from build123d import *

# Parameters (mm, degrees)
F1_R         = 2.5
F2_DEPTH     = 7.5
F3_W         = 3.4
F3_H         = 15.4505071864
F3_W_2       = 3.8797123611
F3_W_3       = 3.8316924378
F4_DEPTH     = 16.41578
F6_DEPTH     = 2.8
F8_DEPTH     = 2.8
F9_R         = 0.1
F10_R        = 2.5
F11_DEPTH    = 7.5
F12_W        = 3
F12_H        = 7.5577301905
F13_DEPTH    = 15.0010001
F14_T1_DEPTH = 16.5892781094
F16_W        = 15
F16_H        = 15
F17_DEPTH    = 30


# Not quite as in the source:
# - a fillet or chamfer that OpenCascade refuses, or shapes differently, is made with other operations: its cross-section is extruded or revolved along the edge and cut away or added


with BuildPart() as f2:
    # F1 (on Right) → F2 (new body, symmetric)
    with BuildSketch(Plane.YZ):
        with BuildLine():
            Line((7.5, -12.5), (7.5, 0))
            ThreePointArc((7.5, 0), (0, 7.5), (-7.5, 0))
            Line((-7.5, 0), (-7.5, -12.5))
            Line((-7.5, -12.5), (7.5, -12.5))
        make_face()
        Circle(F1_R, mode=Mode.SUBTRACT)
    extrude(amount=F2_DEPTH, both=True)

    # F3 (on Front) → F4 (cut, symmetric)
    with BuildSketch(Plane.XZ):
        with Locations((0, 0.7252535932)):
            Rectangle(F3_W, F3_H)
        with Locations((-6.6398561805, 0.7252535932)):
            Rectangle(F3_W_2, F3_H)
        with Locations((6.6158462189, 0.7252535932)):
            Rectangle(F3_W_3, F3_H)
    extrude(amount=F4_DEPTH, both=True, mode=Mode.SUBTRACT)

    # F5 (on face) → F6 (cut, through all)
    with BuildSketch(Plane(origin=(-7.5, 0, 0), x_dir=(0, -1, 0), z_dir=(-1, 0, 0))):
        with BuildLine():
            ThreePointArc((2.6925824036, -7), (6.1824092402, -4.2459175671), (7.5, 0))
            ThreePointArc((7.5, 0), (-4.2459175671, 6.1824092402), (-2.6925824036, -7))
            Line((-2.6925824036, -7), (2.6925824036, -7))
        make_face()
        with BuildLine():
            Line((2.6925824036, -7), (-2.6925824036, -7))
            ThreePointArc((-2.6925824036, -7), (0, -7.5), (2.6925824036, -7))
        make_face()
    extrude(amount=-F6_DEPTH, mode=Mode.SUBTRACT)

    # F7 (on face) → F8 (cut, through all)
    with BuildSketch(Plane.YZ.offset(7.5)):
        with BuildLine():
            Line((2.6925824036, -7), (-2.6925824036, -7))
            ThreePointArc((-2.6925824036, -7), (0, -7.5), (2.6925824036, -7))
        make_face()
        with BuildLine():
            ThreePointArc((2.6925824036, -7), (6.1824092402, -4.2459175671), (7.5, 0))
            ThreePointArc((7.5, 0), (-4.2459175671, 6.1824092402), (-2.6925824036, -7))
            Line((-2.6925824036, -7), (2.6925824036, -7))
        make_face()
    extrude(amount=-F8_DEPTH, mode=Mode.SUBTRACT)

    # F9
    f9_edges = [f2.edges().sort_by_distance(p)[0] for p in [
        (7.5, -5.096291, -7),
        (7.5, 0, -7.5),
        (7.5, 5.096291, -7),
        (-7.5, 5.096291, -7),
        (-7.5, 0, -7.5),
        (-7.5, -5.096291, -7),
    ]]
    fillet(f9_edges, radius=F9_R)

    # F16 (on face) → F17 (join)
    with BuildSketch(Plane(origin=(0, 0, -12.5), x_dir=(1, 0, 0), z_dir=(0, 0, -1))):
        Rectangle(F16_W, F16_H)
    extrude(amount=F17_DEPTH)

    # F18: F2 across face


with BuildPart() as f11:
    # F10 (on Right) → F11 (new body, symmetric)
    with BuildSketch(Plane.YZ):
        with BuildLine():
            Line((-7.5, 15.0892781094), (-7.5, 0))
            ThreePointArc((-7.5, 0), (0, -7.5), (7.5, 0))
            Line((7.5, 0), (7.5, 15.0892781094))
            Line((7.5, 15.0892781094), (-7.5, 15.0892781094))
        make_face()
        Circle(F10_R, mode=Mode.SUBTRACT)
    extrude(amount=F11_DEPTH, both=True)

    # F12 (on face) → F13 (cut, through all)
    with BuildSketch(Plane.XZ.offset(7.5)):
        with Locations((-3.2, 3.7788650952)):
            Rectangle(F12_W, F12_H)
        with Locations((3.2, 3.7788650952)):
            Rectangle(F12_W, F12_H)
    extrude(amount=-F13_DEPTH, mode=Mode.SUBTRACT)

    # F14: fillet of radius 0.1 on 4 edges, made by hand

    # F14_s2 → F14_t1 (cut)
    with BuildSketch(Plane.XY.offset(-1.25)):
        with BuildLine():
            ThreePointArc((-7.4, 7.5), (-7.4707106781, 7.4707106781), (-7.5, 7.4))
            Line((-7.5, 7.4), (-7.5, 7.5))
            Line((-7.5, 7.5), (-7.4, 7.5))
        make_face()
        with BuildLine():
            ThreePointArc((-7.5, -7.4), (-7.4707106781, -7.4707106781), (-7.4, -7.5))
            Line((-7.4, -7.5), (-7.5, -7.5))
            Line((-7.5, -7.5), (-7.5, -7.4))
        make_face()
        with BuildLine():
            ThreePointArc((7.4, 7.5), (7.4707106781, 7.4707106781), (7.5, 7.4))
            Line((7.5, 7.4), (7.5, 7.5))
            Line((7.5, 7.5), (7.4, 7.5))
        make_face()
        with BuildLine():
            ThreePointArc((7.5, -7.4), (7.4707106781, -7.4707106781), (7.4, -7.5))
            Line((7.4, -7.5), (7.5, -7.5))
            Line((7.5, -7.5), (7.5, -7.4))
        make_face()
    extrude(amount=F14_T1_DEPTH, mode=Mode.SUBTRACT)


with BuildPart() as f2_1:
    add(f2.part)
    add(f2.part.mirror(Plane(origin=(0, 0, -42.5), x_dir=(1, 0, 0), z_dir=(0, 0, -1))))


solid = f2_1.part
Work out the finished part from the listing and answer in its coordinate system (mm). A direction names the side the tool comes from. Round coordinates to 2 decimals unless told otherwise and drop trailing zeros. Write each loop counter-clockwise with the first axis right and the second up, starting at its lowest first coordinate (ties: lowest second). Pieces come first, ordered by that corner, then holes. Notation, with made-up numbers: (-38.5, 38.5) - (7.5, 38.5) arc R17 ccw to (7.5, 62.5) - close; hole circle Ø7 at (-18, -34). An arc over 180 degrees is marked (long way). Answer in a Markdown table with one row per item. Add a question column.
1. A cutting plane is placed at D-D, the plane y = 0. Count the separate pieces of the cut face and the enclosed holes in it, and give its area (3 significant figures).
2. The mould has two halves that part along Y. Classify faces 4 (the cylindrical face through (-3.18, 0.16, 7.5)), 5 (the flat face through (7.5, 0, -43)), 6 (the cylindrical face through (-3.22, -0.54, -2.44)): +Y half, -Y half, draft (parallel to the pull), parting line (faces both ways), or undercut.
3. For faces 1 (the flat face through (-6, 5, -78)), 2 (the cylindrical face through (6.1, 0, -77.5)), 3 (the flat face through (6, 5, -78)), determine the directions among +Z, -Z, +X, -X, +Y, -Y from which every point of the face is accessible in a straight line to the end or side of a thin tool.
4. A cutting plane is placed at A-A, the plane z = -5.5. Determine the outline of the cut face in (x, y).
5. Given pin 1 (5 mm diameter, centred on x = 6, y = 5.5, fed in from -Z); pin 2 (3 mm diameter, centred on x = -6, y = -5, fed in from +Z); pin 3 (0.8 mm diameter, centred on x = 5.5, y = 5.5, fed in from +Z), each flat-ended and moving along its own axis, determine where each tip first touches the part or whether it passes through.
6. A cutting plane is placed at C-C, the plane x = -3.25. Determine the outline of the cut face in (y, z).
7. Find the intervals of material crossed by line 1 along Z through (x, y) = (-4, 0); line 2 along X through (y, z) = (1.5, -80); line 3 along Z through (x, y) = (3.75, -6.25), in increasing order. Write a range as from..to.
8. A cutting plane is placed at B-B, the plane z = -84. Determine the outline of the cut face in (x, y).
Worked out:
| question | item | result |
|---|---|---|
| 1 | separate pieces | 5 |
| 1 | enclosed holes | 0 |
| 1 | area | 1,170 mm^2 |
| 2 | face 4 | parting line |
| 2 | face 5 | draft |
| 2 | face 6 | undercut |
| 3 | face 1 | -Z, -X, +Y, -Y |
| 3 | face 2 | -Z, +X |
| 3 | face 3 | -Z, +X, +Y, -Y |
| 4 | outline | (-4.7, -7.5) - (-1.7, -7.5) - (-1.7, 7.5) - (-4.7, 7.5) - close; (1.7, -7.5) - (4.7, -7.5) - (4.7, 7.5) - (1.7, 7.5) - close |
| 5 | pin 1 | z = -91.7 |
| 5 | pin 2 | z = 6.18 |
| 5 | pin 3 | z = -7 |
| 6 | outline | (-7.5, -85) arc R7.5 ccw to (7.5, -85) - (7.5, 0) arc R7.5 ccw to (-7.5, 0) - close; hole circle Ø5 at (0, -85); hole circle Ø5 at (0, 0) |
| 7 | line 1 | -92.5..-87.5, -82.5..-2.5, 2.5..7.5 |
| 7 | line 2 | -4.7..-1.7, 1.7..4.7 |
| 7 | line 3 | -89.15..4.15 |
| 8 | outline | (-4.7, -7.5) - (-1.7, -7.5) - (-1.7, -2.29) - (-4.7, -2.29) - close; (-4.7, 2.29) - (-1.7, 2.29) - (-1.7, 7.5) - (-4.7, 7.5) - close; (1.7, -7.5) - (4.7, -7.5) - (4.7, -2.29) - (1.7, -2.29) - close; (1.7, 2.29) - (4.7, 2.29) - (4.7, 7.5) - (1.7, 7.5) - close |
